```python
from build123d import *

# Parameters (mm, degrees)
SKETCH1_R             = 15
BOSS_EXTRUDE1_DEPTH   = 10
SKETCH1_R_2           = 10
BOSS_EXTRUDE1_2_DEPTH = 10
BOSS_EXTRUDE3_DEPTH   = 10
SKETCH13_R            = 4
CUT_EXTRUDE1_DEPTH    = 20
BOSS_EXTRUDE7_START   = 2.5
SKETCH14_R            = 15
SKETCH14_R_2          = 4
BOSS_EXTRUDE7_DEPTH   = 2.5
SKETCH15_R            = 4
BOSS_EXTRUDE8_DEPTH   = 2
ECHELLE1_SCALE        = 0.6


with BuildPart() as part:
    # Sketch1 → Boss-Extrude1 (new body)
    with BuildSketch(Plane.XY):
        Circle(SKETCH1_R)
    extrude(amount=BOSS_EXTRUDE1_DEPTH)



with BuildPart() as body_2:
    # Sketch1 → Boss-Extrude1 2 (new body)
    with BuildSketch(Plane.XY):
        with Locations((300, 0)):
            Circle(SKETCH1_R_2)
    extrude(amount=BOSS_EXTRUDE1_2_DEPTH)


with BuildPart() as part_1:
    add(part.part)

    add(body_2.part)  # Boss-Extrude3 merges body 2
    # Sketch5 → Boss-Extrude3 (add)
    with BuildSketch(Plane.XY):
        with BuildLine():
            Line((300, 10), (11.180339887, 10))
            ThreePointArc((11.180339887, 10), (14.012585384, 5.352331347), (15, 0))
            ThreePointArc((15, 0), (14.012585384, -5.352331347), (11.180339887, -10))
            Line((11.180339887, -10), (300, -10))
            ThreePointArc((300, -10), (290, 0), (300, 10))
        make_face()
    extrude(amount=BOSS_EXTRUDE3_DEPTH)

    # Sketch13 → Cut-Extrude1 (cut)
    with BuildSketch(Plane(origin=(0, 0, 0), x_dir=(-1, 0, 0), z_dir=(0, 0, -1))):
        with Locations((-300, 0)):
            Circle(SKETCH13_R)
        Circle(SKETCH13_R)
    extrude(amount=-CUT_EXTRUDE1_DEPTH, mode=Mode.SUBTRACT)

    # Sketch14 → Boss-Extrude7 (add)
    with BuildSketch(Plane(origin=(0, 0, 0), x_dir=(-1, 0, 0), z_dir=(0, 0, -1)).offset(BOSS_EXTRUDE7_START)):
        Circle(SKETCH14_R)
        Circle(SKETCH14_R_2, mode=Mode.SUBTRACT)
    extrude(amount=-BOSS_EXTRUDE7_DEPTH)

    # Sketch15 → Boss-Extrude8 (add)
    with BuildSketch(Plane.XY.offset(10)):
        with BuildLine():
            ThreePointArc((300, 10), (290, 0), (300, -10))
            ThreePointArc((300, -10), (307.071067812, -7.071067812), (310, 0))
            ThreePointArc((310, 0), (307.071067812, 7.071067812), (300, 10))
        make_face()
        with Locations(Location((300, 0, 0), (0, 0, 180))):
            Circle(SKETCH15_R, mode=Mode.SUBTRACT)
    extrude(amount=BOSS_EXTRUDE8_DEPTH)


with BuildPart() as part_2:
    # Echelle1: scaled about (141.196241325, 0, 4.894209778)
    add(part_1.part.scale(ECHELLE1_SCALE).moved(Location((56.47849653, 0, 1.957683911))))


solid = part_2.part
```
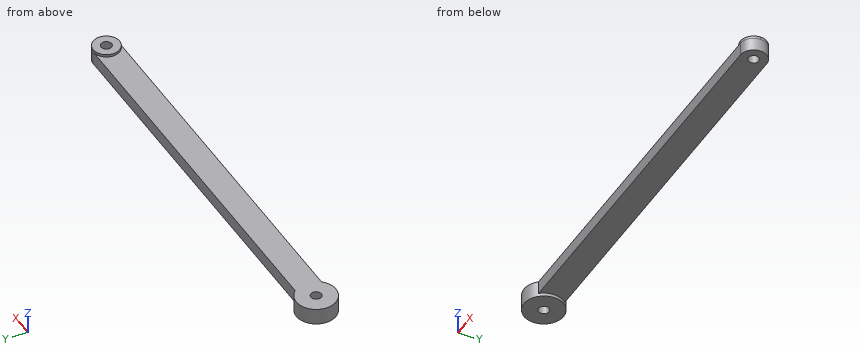
Here's how the part is built. I have some questions about the finished solid (model axes, mm). Coordinates: 2 decimals unless noted, no trailing zeros. Order: outer loops, then holes, each group sorted by start corner. A loop starts at its lowest first (then second) coordinate and runs counter-clockwise, first axis right, second up. Notation, with made-up numbers: (46, 50.25) - (58, 50.25) arc R27 ccw to (58, 71.25) - close; hole circle Ø4 at (67, -14.5). An arc over 180 degrees is marked (long way). One line per question, with ' | ' between items. Start each with the question number.
1. Please list where these lines run through material, in increasing order: line 1 along X through (y, z) = (1, 4); line 2 along Z through (x, y) = (173, 1.5); line 3 along Y through (x, z) = (191, 4.75). Write a range as [from, to].
2. If we section it at A-A (z = 6.25): Write out the boundary of the cut face in (x, y).
3. I'm going to push flat-ended pins straight in: pin 1 Ø4 at (y, z) = (-3, 7.5) entering from +X; pin 2 Ø5 at (x, z) = (130.5, 4.5) entering from +Y; pin 3 Ø1 at (y, z) = (3.5, 4.5) entering from -X. Where does each tip first touch, or does it pass through?
4. If we section it at B-B (x = 224.5): Write out the boundary of the cut face in (y, z), and give its area (3 significant figures).
Model answer:
1) line 1: x = [47.53, 54.3], [58.66, 234.3], [238.66, 242.39] | line 2: z = [1.96, 7.96] | line 3: y = [-6, 6]
2) outline: (63.19, -6) - (236.48, -6) arc R6 ccw to (236.48, 6) - (63.19, 6) arc R9 ccw (long way) to start; hole circle Ø4.8 at (56.48, 0); hole circle Ø4.8 at (236.48, 0)
3) pin 1: stops at x = 242.39 | pin 2: stops at y = 6 | pin 3: stops at x = 47.99
4) outline: (-6, 1.96) - (6, 1.96) - (6, 7.96) - (-6, 7.96) - close | area: 72.0 mm²
